The model under review builds one solid part; all positions refer to its coordinate system, in mm. Face numbers are marked on the shaded views. A direction names the side the tool comes from. Give positions to 0.01 mm unless a question says otherwise; leave off trailing zeros. Loops run counter-clockwise (first coordinate to the right, second up) from the corner with the lowest first, then second, coordinate; pieces in that order, holes last. Notation, with made-up numbers: M -37.5,-19 L -27.5,-19 A30 ccw -27.5,20 Z; hole C -4.5,88.5 d2. An arc over 180 degrees is marked long. Return JSON: item names as keys, results as strings.
```python
from build123d import *

# Parameters (mm, degrees)
SKETCH1_R           = 1.6
SKETCH1_W           = 21
SKETCH1_H           = 41
BOSS_EXTRUDE1_DEPTH = 11
SKETCH6_W           = 21
SKETCH6_H           = 0.1
CUT_EXTRUDE1_DEPTH  = 91.428148273
SKETCH7_W           = 21
SKETCH7_H           = 41.2
SKETCH7_R           = 1.6
CUT_EXTRUDE2_DEPTH  = 11
SKETCH8_R           = 1.95
CUT_EXTRUDE3_DEPTH  = 11


with BuildPart() as part:
    # Sketch1 → Boss-Extrude1 (new body)
    with BuildSketch(Plane.XY):
        with BuildLine():
            Line((-20, 70), (-20, -50))
            ThreePointArc((-20, -50), (-2.5, -67.5), (15, -50))
            Line((15, -50), (15, 70))
            ThreePointArc((15, 70), (-2.5, 87.5), (-20, 70))
        make_face()
        with Locations((-7.5, 79.5)):
            Circle(SKETCH1_R, mode=Mode.SUBTRACT)
        with Locations(Location((2.5, 79.5, 0), (0, 0, 180))):
            Circle(SKETCH1_R, mode=Mode.SUBTRACT)
        with Locations((2.5, 30.5)):
            Circle(SKETCH1_R, mode=Mode.SUBTRACT)
        with Locations(Location((-7.5, 30.5, 0), (0, 0, 180))):
            Circle(SKETCH1_R, mode=Mode.SUBTRACT)
        with Locations((-2.5, 55)):
            Rectangle(SKETCH1_W, SKETCH1_H, mode=Mode.SUBTRACT)
    extrude(amount=BOSS_EXTRUDE1_DEPTH)

    # Sketch6 → Cut-Extrude1 (cut, through all)
    with BuildSketch(Plane.XY.offset(11)):
        with Locations((-2.5, 75.55)):
            Rectangle(SKETCH6_W, SKETCH6_H)
        with Locations((-2.5, 34.45)):
            Rectangle(SKETCH6_W, SKETCH6_H)
    extrude(amount=-CUT_EXTRUDE1_DEPTH, mode=Mode.SUBTRACT)

    # Sketch7 → Cut-Extrude2 (cut)
    with BuildSketch(Plane(origin=(0, 0, 0), x_dir=(-1, 0, 0), z_dir=(0, 0, -1))):
        with Locations((2.5, -35)):
            Rectangle(SKETCH7_W, SKETCH7_H)
        with Locations((-2.5, -10.5)):
            Circle(SKETCH7_R)
        with Locations((7.5, -10.5)):
            Circle(SKETCH7_R)
        with Locations((-2.5, -59.5)):
            Circle(SKETCH7_R)
        with Locations((7.5, -59.5)):
            Circle(SKETCH7_R)
    extrude(amount=-CUT_EXTRUDE2_DEPTH, mode=Mode.SUBTRACT)

    # Sketch8 → Cut-Extrude3 (cut)
    with BuildSketch(Plane.XY.offset(11)):
        with Locations((-7.5, 79.5)):
            Circle(SKETCH8_R)
        with Locations((2.5, 79.5)):
            Circle(SKETCH8_R)
        with Locations((2.5, 30.5)):
            Circle(SKETCH8_R)
        with Locations((-7.5, 30.5)):
            Circle(SKETCH8_R)
        with Locations((2.5, -10.5)):
            Circle(SKETCH8_R)
        with Locations((-7.5, -10.5)):
            Circle(SKETCH8_R)
        with Locations((2.5, -59.5)):
            Circle(SKETCH8_R)
        with Locations((-7.5, -59.5)):
            Circle(SKETCH8_R)
    extrude(amount=-CUT_EXTRUDE3_DEPTH, mode=Mode.SUBTRACT)


solid = part.part
```
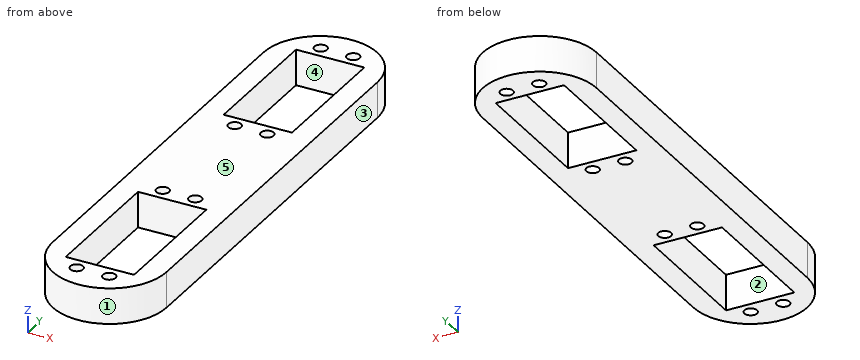
1) The part is to be moulded in two halves that separate along X. For the marked faces 1, 2 and 3, say which applies: released by +X, released by -X, zero draft, split by the parting line, or undercut.
From the geometry:
{"face 1": "split by the parting line", "face 2": "undercut", "face 3": "released by +X"}
2) Wall thickness on L1, parallel to Y at x = 6.5, z = 9; L2, parallel to Y at x = -10.5, z = 6.5; L3, parallel to X at y = 62, z = 2: over which ranges is each line inside the solid? List them lowest first. Write a range as from..to.
From the geometry:
{"L1": "-65.01..-55.6, -14.4..34.4, 75.6..85.01", "L2": "-65.56..-55.6, -14.4..34.4, 75.6..85.56", "L3": "-20..-13, 8..15"}
3) Consider section A-A on y = 30.5. Write out the cut boundary in (x, z), then the cut area to 3 significant figures.
From the geometry:
{"outline": "M -20,0 L -9.45,0 L -9.45,11 L -20,11 Z; M -5.55,0 L 0.55,0 L 0.55,11 L -5.55,11 Z; M 4.45,0 L 15,0 L 15,11 L 4.45,11 Z", "area": "299 mm²"}
4) Consider section D-D on x = 2.5. Write out the cut boundary in (y, z).
From the geometry:
{"outline": "M -66.77,0 L -61.45,0 L -61.45,11 L -66.77,11 Z; M -57.55,0 L -55.6,0 L -55.6,11 L -57.55,11 Z; M -14.4,0 L -12.45,0 L -12.45,11 L -14.4,11 Z; M -8.55,0 L 28.55,0 L 28.55,11 L -8.55,11 Z; M 32.45,0 L 34.4,0 L 34.4,11 L 32.45,11 Z; M 75.6,0 L 77.55,0 L 77.55,11 L 75.6,11 Z; M 81.45,0 L 86.77,0 L 86.77,11 L 81.45,11 Z"}
5) Tool access review of the marked faces 4 and 5: name each direction out of +Z, -Z, +X, -X, +Y, -Y from which nothing blocks a thin tool from reaching the whole face with its end or side.
From the geometry:
{"face 4": "+Z, -Z", "face 5": "+Z, +X, -X, +Y, -Y"}
6) Insertion check: pin 1 (1 mm diameter, centred on x = -16, z = 9, fed in from -Y). The pin has a flat end and moves straight along its axis. Give the tip position at first contact, or say it passes through.
From the geometry:
{"pin 1": "y = -61.72"}
7) Consider section B-B on y = 57.5. Write out the cut boundary in (x, z).
From the geometry:
{"outline": "M -20,0 L -13,0 L -13,11 L -20,11 Z; M 8,0 L 15,0 L 15,11 L 8,11 Z"}
8) Consider section C-C on z = 4.75. Count the separate pieces of the cut face and the enclosed holes in it, then the cut area to 3 significant figures.
From the geometry:
{"separate pieces": "1", "enclosed holes": "10", "area": "3,340 mm²"}
